Read the model definition and answer for the solid it produces. Units are mm, in the model's axes. A direction names the side the tool comes from. Coordinates: 2 decimals unless noted, no trailing zeros. Loops run counter-clockwise (first coordinate to the right, second up) from the corner with the lowest first, then second, coordinate; pieces in that order, holes last. Notation, with made-up numbers: (44, -26) - (63, -26) arc R22 ccw to (63, 0) - close; hole circle Ø4 at (-4, 80.5). An arc over 180 degrees is marked (long way). One line per item, written item: value. Start each with the question number.
from build123d import *

# Parameters (mm, degrees)
SKETCH4_W           = 114.3
SKETCH4_H           = 76.2
BOSS_EXTRUDE2_DEPTH = 25.4
CUT_EXTRUDE1_REACH  = 47.72
SKETCH5_W           = 107.95
SKETCH5_H           = 69.85
SKETCH6_R           = 2.54
BOSS_EXTRUDE3_DEPTH = 25.4


with BuildPart() as part:
    # Sketch4 → Boss-Extrude2 (new body, symmetric)
    with BuildSketch(Plane(origin=(0, 0, 0), x_dir=(1, 0, 0), z_dir=(0, 1, 0))):
        Rectangle(SKETCH4_W, SKETCH4_H)
    extrude(amount=BOSS_EXTRUDE2_DEPTH, both=True)

    # Sketch5 → Cut-Extrude1 (cut, up to next)
    with BuildSketch(Plane(origin=(0, -20.32, 0), x_dir=(-1, 0, 0), z_dir=(0, -1, 0)), mode=Mode.PRIVATE) as cut_extrude1_sk1:
        Rectangle(SKETCH5_W, SKETCH5_H)
    cut_extrude1_tool1 = extrude(cut_extrude1_sk1.sketch, amount=-CUT_EXTRUDE1_REACH, mode=Mode.PRIVATE) & part.part
    add(cut_extrude1_tool1.solids().sort_by_distance((0, -20.32, 0))[0], mode=Mode.SUBTRACT)

    # Sketch6 → Boss-Extrude3 (add, symmetric)
    with BuildSketch(Plane(origin=(0, 0, 0), x_dir=(1, 0, 0), z_dir=(0, 1, 0))):
        with Locations((34.29, 17.78)):
            Circle(SKETCH6_R)
        with Locations((34.29, -15.24)):
            Circle(SKETCH6_R)
        with Locations((0, -15.24)):
            Circle(SKETCH6_R)
        with Locations((-34.29, -15.24)):
            Circle(SKETCH6_R)
        with Locations((-34.29, 17.78)):
            Circle(SKETCH6_R)
    extrude(amount=BOSS_EXTRUDE3_DEPTH, both=True)


solid = part.part
1) For faces 1 (the cylindrical face through (32.3, 2.9, -16.2)), 2 (the flat face through (-34, 25.4, 15)), determine the directions among +Z, -Z, +X, -X, +Y, -Y from which every point of the face is accessible in a straight line to the end or side of a thin tool.
2) Determine the mould class of faces 3 (the flat face through (-1, 0, 38.1)), 4 (the flat face through (-57.15, 0, 1)), 5 (the flat face through (53.975, 2, 0)) for opening direction X: released by +X, released by -X, zero draft, split by the parting line, or undercut.
3) Straight lines are drawn through the part: L1, parallel to X at y = -5, z = -18 (3 decimals); L2, parallel to Z at x = -5, y = -20 (3 decimals); L3, parallel to X at y = -7, z = -26 (3 decimals). For each, find the intervals that lie inside material, in ascending order.
4) A flat-ended cylindrical pin translates along its axis: P1, Ø3, axis at x = 7.5, z = -26, coming from the +Y side. Find the tip coordinate at first contact, or state that the pin passes through.
5) Section C-C, the plane z = -17.78 is taken. Determine the outline of the cut face in (x, y) (3 decimals).
6) Section A-A, the plane y = -1 is taken. Determine the outline of the cut face in (x, z) (3 decimals), and give its area (3 significant figures).
7) Section B-B, the plane x = 0 is taken. Determine the outline of the cut face in (y, z) (3 decimals), and give its area (3 significant figures).
8) Section D-D, the plane z = -2 is taken. Determine the outline of the cut face in (x, y) (3 decimals), and give its area (3 significant figures).
Answer below:
1. face 1: +Y
1. face 2: +Z, -Z, +X, -X, +Y
2. face 3: zero draft
2. face 4: released by -X
2. face 5: undercut
3. L1: -57.15 to -53.975, -36.82 to -31.76, 31.76 to 36.82, 53.975 to 57.15
3. L2: -38.1 to -34.925, 34.925 to 38.1
3. L3: -57.15 to -53.975, 53.975 to 57.15
4. P1: y = -20.32
5. outline: (-57.15, -25.4) - (57.15, -25.4) - (57.15, 25.4) - (53.975, 25.4) - (53.975, -20.32) - (36.83, -20.32) - (36.83, 25.4) - (31.75, 25.4) - (31.75, -20.32) - (-31.75, -20.32) - (-31.75, 25.4) - (-36.83, 25.4) - (-36.83, -20.32) - (-53.975, -20.32) - (-53.975, 25.4) - (-57.15, 25.4) - close
6. outline: (-57.15, -38.1) - (57.15, -38.1) - (57.15, 38.1) - (-57.15, 38.1) - close; circle Ø5.08 at (-34.29, -17.78); circle Ø5.08 at (-34.29, 15.24); circle Ø5.08 at (0, 15.24); circle Ø5.08 at (34.29, -17.78); circle Ø5.08 at (34.29, 15.24); hole (-53.975, -34.925) - (53.975, -34.925) - (53.975, 34.925) - (-53.975, 34.925) - close
6. area: 1,270 mm2
7. outline: (-25.4, -38.1) - (25.4, -38.1) - (25.4, -34.925) - (-20.32, -34.925) - (-20.32, 12.7) - (25.4, 12.7) - (25.4, 17.78) - (-20.32, 17.78) - (-20.32, 34.925) - (25.4, 34.925) - (25.4, 38.1) - (-25.4, 38.1) - close
7. area: 910 mm2
8. outline: (-57.15, -25.4) - (57.15, -25.4) - (57.15, 25.4) - (53.975, 25.4) - (53.975, -20.32) - (-53.975, -20.32) - (-53.975, 25.4) - (-57.15, 25.4) - close
8. area: 871 mm2
